Part print with two shaded views. Sizes in mm from the minimum x, y, z corner. A direction names the side the tool comes from. Round coordinates to 2 decimals unless told otherwise and drop trailing zeros. Order: outer loops, then holes, each group sorted by start corner. A loop starts at its lowest first (then second) coordinate and runs counter-clockwise, first axis right, second up. Notation, with made-up numbers: (-26.5, 75.5) -> (21.5, 75.5) arc R29 ccw to (21.5, 101.5) -> close; hole circle Ø8 at (-1.5, 61.5). An arc over 180 degrees is marked (long way). Put each result on its own line as item: value. Start each with the question number.
Q1. Cut at C-C, the plane z = 39. List the corners of the cut face in (x, y).
Q2. Probe L1, parallel to Z at x = 11, y = 10 (1 decimal); L2, parallel to X at y = 7.5, z = 93; L3, parallel to Y at x = 8, z = 93.5. List the from-to ranges inside material, lowest first.
Q3. Cut at D-D, the plane x = 22.5. List the corners of the cut face in (y, z).
Q4. Cut at B-B, the plane y = 14. List the corners of the cut face in (x, z) (1 decimal).
Q5. Pull direction X, two halves, no side cores. Call the marked faces 3, 4 and 5: released by +X, released by -X, zero draft, split by the parting line, or undercut.
Q6. Cut at A-A, the plane z = 71. List the corners of the cut face in (x, y), and give its area (3 significant figures).
Q7. Flat gauge pins, fed straight in: P1, Ø4, axis at x = 41.5, z = 36.5, coming from the +Y side; P2, Ø7, axis at x = 32, y = 7.5, coming from the -Z side; P3, Ø1, axis at x = 51, y = 15.5, coming from the +Z side (1 decimal); P4, Ø6, axis at x = 31, y = 17, coming from the -Z side. Where does each tip first touch, or does it go through?
Q8. 3-axis set-ups, long thin cutter, end or side, ignore diameter. For the marked faces 1 and 2: which of +Z, -Z, +X, -X, +Y, -Y reach the whole face in a straight line?
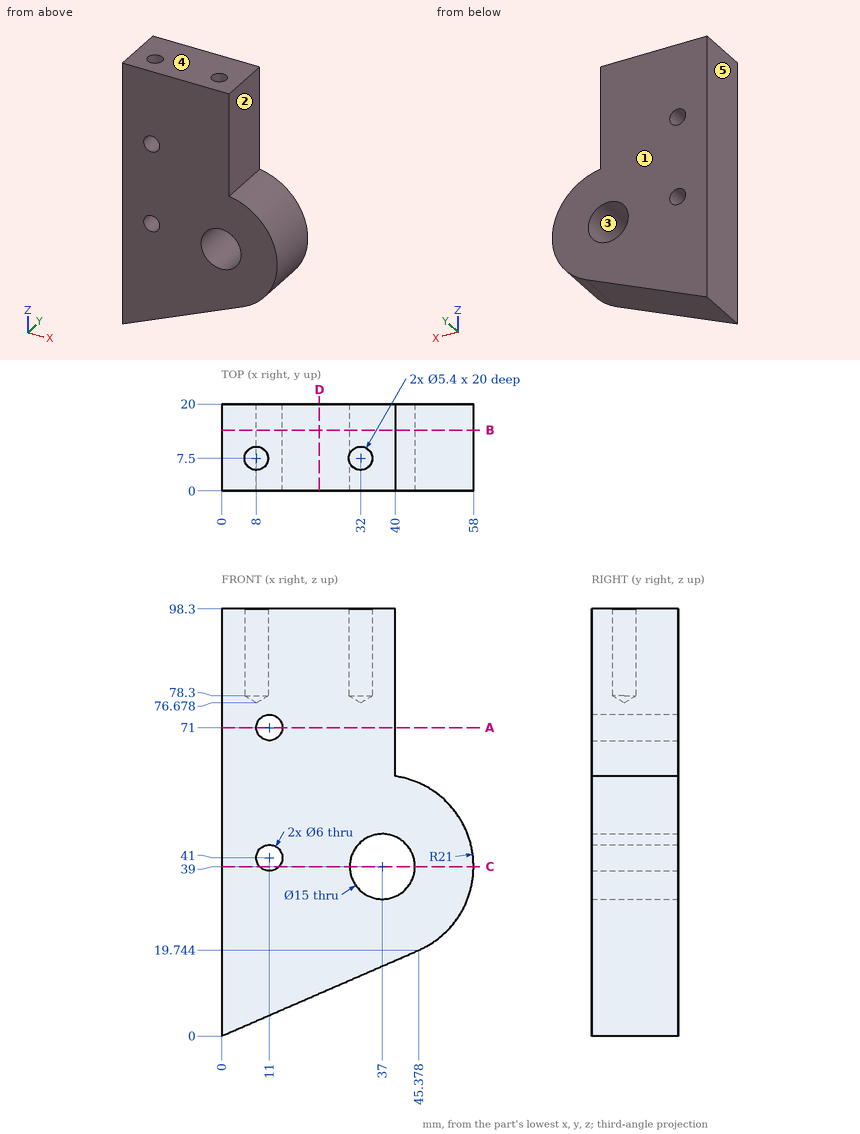
Ans:
1. outline: (0, 0) -> (8.76, 0) -> (8.76, 20) -> (0, 20) -> close; (13.24, 0) -> (29.5, 0) -> (29.5, 20) -> (13.24, 20) -> close; (44.5, 0) -> (58, 0) -> (58, 20) -> (44.5, 20) -> close
2. L1: z = 4.8 to 38, 44 to 68, 74 to 98.3
2. L2: x = 0 to 5.3, 10.7 to 29.3, 34.7 to 40
2. L3: y = 0 to 4.8, 10.2 to 20
3. outline: (0, 9.79) -> (20, 9.79) -> (20, 98.3) -> (0, 98.3) -> close
4. outline: (0, 0) -> (45.4, 19.7) arc R21 ccw to (40, 59.8) -> (40, 98.3) -> (0, 98.3) -> close; hole circle Ø6 at (11, 41); hole circle Ø6 at (11, 71); hole circle Ø15 at (37, 39)
5. face 3: undercut
5. face 4: zero draft
5. face 5: released by -X
6. outline: (0, 0) -> (8, 0) -> (8, 20) -> (0, 20) -> close; (14, 0) -> (40, 0) -> (40, 20) -> (14, 20) -> close
6. area: 680 mm^2
7. P1: passes through
7. P2: stops at z = 12.4
7. P3: stops at z = 55.1
7. P4: stops at z = 12.18
8. face 1: +Z, -Z, +X, -X, +Y
8. face 2: +Z, +X, +Y, -Y
